Verification items for the finished model (mm, model axes). A direction names the side the tool comes from. Round coordinates to 2 decimals unless told otherwise and drop trailing zeros. Order: outer loops, then holes, each group sorted by start corner. A loop starts at its lowest first (then second) coordinate and runs counter-clockwise, first axis right, second up. Notation, with made-up numbers: (-31, -34) -> (15, -34) arc R14 cw to (15, -24) -> close; hole circle Ø4 at (36, 37). An arc over 180 degrees is marked (long way). Put each result on its own line as item: value.
```python
from build123d import *

# Parameters (mm, degrees)
BOSS_EXTRU_1_DEPTH      = 5
BOSS_EXTRU_1_2_DEPTH    = 5
BOSS_EXTRU_1_3_DEPTH    = 5
BOSS_EXTRU_1_4_DEPTH    = 5
BOSS_EXTRU_2_DEPTH      = 3
ENL_V_MAT_EXTRU_2_DEPTH = 186.027362841
ESQUISSE4_R             = 1.6
BOSS_EXTRU_3_DEPTH      = 3
BOSS_EXTRU_4_DEPTH      = 183.014563107
BOSS_EXTRU_6_DEPTH      = 169.006591337
BOSS_EXTRU_7_DEPTH      = 174.257281553
BOSS_EXTRU_8_DEPTH      = 177.5
ESQUISSE10_R            = 28
BOSS_EXTRU_9_DEPTH      = 2
BOSS_EXTRU_11_START     = 2.5
ESQUISSE11_W            = 257.5
ESQUISSE11_H            = 265.5
ESQUISSE11_R            = 28
BOSS_EXTRU_11_DEPTH     = 2.5
ESQUISSE12_R            = 2.1
BOSS_EXTRU_12_DEPTH     = 10.5
ESQUISSE13_R            = 5.1
ENL_V_MAT_EXTRU_3_DEPTH = 5
BOSS_EXTRU_13_DEPTH     = 10.5
ESQUISSE15_R            = 5.1
ENL_V_MAT_EXTRU_4_DEPTH = 5
CONG_1_R                = 1


with BuildPart() as part:
    # Esquisse1 → Boss.-Extru.1 (new body)
    with BuildSketch(Plane.XY):
        Polygon((128.75, -132.75), (88.75, -132.75), (88.75, -111.507281553), (108.75, -91.507281553), (128.75, -91.507281553), align=None)
    extrude(amount=BOSS_EXTRU_1_DEPTH)



with BuildPart() as body_2:
    # Esquisse1 → Boss.-Extru.1 2 (new body)
    with BuildSketch(Plane.XY):
        Polygon((128.75, 132.75), (80.256591337, 132.75), (80.256591337, 102.75), (100.256591337, 82.75), (128.75, 82.75), align=None)
    extrude(amount=BOSS_EXTRU_1_2_DEPTH)


with BuildPart() as body_3:
    # Esquisse1 → Boss.-Extru.1 3 (new body)
    with BuildSketch(Plane.XY):
        Polygon((-128.75, -132.75), (-128.75, -91.507281553), (-108.75, -91.507281553), (-88.75, -111.507281553), (-88.75, -132.75), align=None)
    extrude(amount=BOSS_EXTRU_1_3_DEPTH)


with BuildPart() as body_4:
    # Esquisse1 → Boss.-Extru.1 4 (new body)
    with BuildSketch(Plane.XY):
        Polygon((-88.75, 132.75), (-88.75, 111.507281553), (-108.75, 91.507281553), (-128.75, 91.507281553), (-128.75, 132.75), align=None)
    extrude(amount=BOSS_EXTRU_1_4_DEPTH)


with BuildPart() as part_1:
    add(part.part)

    add(body_2.part)  # Boss.-Extru.2 merges body 2

    add(body_3.part)  # Boss.-Extru.2 merges body 3

    add(body_4.part)  # Boss.-Extru.2 merges body 4
    # Esquisse2 → Boss.-Extru.2 (add)
    with BuildSketch(Plane(origin=(0, 0, 0), x_dir=(-1, 0, 0), z_dir=(0, 0, -1))):
        Polygon((-80.256591337, 127.75), (-80.256591337, 132.75), (-128.75, 132.75), (-128.75, 82.75), (-123.75, 82.75), (-123.75, 127.75), align=None)
        Polygon((-123.75, -127.75), (-88.75, -127.75), (-88.75, -132.75), (-128.75, -132.75), (-128.75, -91.507281553), (-123.75, -91.507281553), align=None)
        Polygon((88.75, -127.75), (88.75, -132.75), (128.75, -132.75), (128.75, -91.507281553), (123.75, -91.507281553), (123.75, -127.75), align=None)
        Polygon((128.75, 132.75), (88.75, 132.75), (88.75, 127.75), (123.75, 127.75), (123.75, 91.507281553), (128.75, 91.507281553), align=None)
    extrude(amount=BOSS_EXTRU_2_DEPTH)

    # Esquisse3 → Enlèv. mat.-Extru.2 (cut, through all)
    with BuildSketch(Plane.XY.offset(3)):
        Polygon((110, 82.75), (110, 110), (80.256591337, 110), (80.256591337, 102.75), (100.256591337, 82.75), align=None)
        Polygon((-90.257281553, 110), (-110, 110), (-110, 91.507281553), (-108.75, 91.507281553), align=None)
        Polygon((-110, -110), (-110, -91.507281553), (-108.75, -91.507281553), (-90.257281553, -110), align=None)
        Polygon((110, -91.507281553), (110, -110), (90.257281553, -110), (108.75, -91.507281553), align=None)
    extrude(amount=-ENL_V_MAT_EXTRU_2_DEPTH, mode=Mode.SUBTRACT)

    # Esquisse4 → Boss.-Extru.3 (add)
    with BuildSketch(Plane(origin=(0, 0, 3), x_dir=(-1, 0, 0), z_dir=(0, 0, -1))):
        with Locations(Location((-107.5, 107.5, 0), (0, 0, 180))):
            Circle(ESQUISSE4_R)
        with Locations((-107.5, -107.5)):
            Circle(ESQUISSE4_R)
        with Locations(Location((107.5, -107.5, 0), (0, 0, 180))):
            Circle(ESQUISSE4_R)
        with Locations(Location((107.5, 107.5, 0), (0, 0, 180))):
            Circle(ESQUISSE4_R)
    extrude(amount=BOSS_EXTRU_3_DEPTH)

    # Esquisse5 → Boss.-Extru.4 (add)
    with BuildSketch(Plane.XZ.offset(-91.507281553)):
        Polygon((-123.75, 0), (-110, 0), (-110, 3), (-108.75, 3), (-108.75, 5), (-128.75, 5), (-128.75, -3), (-123.75, -3), align=None)
    extrude(amount=BOSS_EXTRU_4_DEPTH)

    # Esquisse7 → Boss.-Extru.6 (add)
    with BuildSketch(Plane(origin=(-88.75, 0, 0), x_dir=(0, 0, -1), z_dir=(1, 0, 0))):
        Polygon((0, 111.507281553), (0, 127.75), (3, 127.75), (3, 132.75), (-5, 132.75), (-5, 111.507281553), align=None)
    extrude(amount=BOSS_EXTRU_6_DEPTH)

    # Esquisse8 → Boss.-Extru.7 (add)
    with BuildSketch(Plane(origin=(0, -91.507281553, 0), x_dir=(1, 0, 0), z_dir=(0, 1, 0))):
        Polygon((123.75, 0), (110, 0), (110, -3), (108.75, -3), (108.75, -5), (128.75, -5), (128.75, 3), (123.75, 3), align=None)
    extrude(amount=BOSS_EXTRU_7_DEPTH)

    # Esquisse9 → Boss.-Extru.8 (add)
    with BuildSketch(Plane.ZY.offset(-88.75)):
        Polygon((0, -111.507281553), (0, -127.75), (-3, -127.75), (-3, -132.75), (5, -132.75), (5, -111.507281553), align=None)
    extrude(amount=BOSS_EXTRU_8_DEPTH)

    # Esquisse10 → Boss.-Extru.9 (add)
    with BuildSketch(Plane.XY.offset(5)):
        with BuildLine():
            Line((100.256591337, 82.75), (31.902373727, 14.39578239))
            ThreePointArc((31.902373727, 14.39578239), (34.999858189, -0.099633105), (31.819897219, -14.577178773))
            Line((31.819897219, -14.577178773), (108.75, -91.507281553))
            Line((108.75, -91.507281553), (88.75, -111.507281553))
            Line((88.75, -111.507281553), (10.599223862, -33.356505415))
            ThreePointArc((10.599223862, -33.356505415), (0, -35), (-10.599223862, -33.356505415))
            Line((-10.599223862, -33.356505415), (-88.75, -111.507281553))
            Line((-88.75, -111.507281553), (-108.75, -91.507281553))
            Line((-108.75, -91.507281553), (-31.819897219, -14.577178773))
            ThreePointArc((-31.819897219, -14.577178773), (-35, 0), (-31.819897219, 14.577178773))
            Line((-31.819897219, 14.577178773), (-108.75, 91.507281553))
            Line((-108.75, 91.507281553), (-90.257281553, 110))
            Line((-90.257281553, 110), (-12.823491891, 32.566210337))
            ThreePointArc((-12.823491891, 32.566210337), (-1.075408771, 34.983474613), (10.798967391, 33.292376054))
            Line((10.798967391, 33.292376054), (80.256591337, 102.75))
            Line((80.256591337, 102.75), (100.256591337, 82.75))
        make_face()
        Circle(ESQUISSE10_R, mode=Mode.SUBTRACT)
    extrude(amount=-BOSS_EXTRU_9_DEPTH)

    # Esquisse11 → Boss.-Extru.11 (add)
    with BuildSketch(Plane.XY.offset(5).offset(BOSS_EXTRU_11_START)):
        Rectangle(ESQUISSE11_W, ESQUISSE11_H)
        Circle(ESQUISSE11_R, mode=Mode.SUBTRACT)
        with BuildLine():
            Line((80.256591337, 111.507281553), (80.256591337, 102.75))
            Line((80.256591337, 102.75), (10.798967391, 33.292376054))
            ThreePointArc((10.798967391, 33.292376054), (-1.075408771, 34.983474613), (-12.823491891, 32.566210337))
            Line((-12.823491891, 32.566210337), (-90.257281553, 110))
            Line((-90.257281553, 110), (-88.75, 111.507281553))
            Line((-88.75, 111.507281553), (80.256591337, 111.507281553))
        make_face(mode=Mode.SUBTRACT)
        with BuildLine():
            Line((-108.75, 91.507281553), (-31.819897219, 14.577178773))
            ThreePointArc((-31.819897219, 14.577178773), (-35, 0), (-31.819897219, -14.577178773))
            Line((-31.819897219, -14.577178773), (-108.75, -91.507281553))
            Line((-108.75, -91.507281553), (-108.75, 91.507281553))
        make_face(mode=Mode.SUBTRACT)
        with BuildLine():
            Line((-88.75, -111.507281553), (-10.599223862, -33.356505415))
            ThreePointArc((-10.599223862, -33.356505415), (0, -35), (10.599223862, -33.356505415))
            Line((10.599223862, -33.356505415), (88.75, -111.507281553))
            Line((88.75, -111.507281553), (-88.75, -111.507281553))
        make_face(mode=Mode.SUBTRACT)
        with BuildLine():
            Line((108.75, -91.507281553), (31.819897219, -14.577178773))
            ThreePointArc((31.819897219, -14.577178773), (34.999858189, -0.099633105), (31.902373727, 14.39578239))
            Line((31.902373727, 14.39578239), (100.256591337, 82.75))
            Line((100.256591337, 82.75), (108.75, 82.75))
            Line((108.75, 82.75), (108.75, -91.507281553))
        make_face(mode=Mode.SUBTRACT)
    extrude(amount=-BOSS_EXTRU_11_DEPTH)

    # Esquisse12 → Boss.-Extru.12 (add)
    # profile 1 of 2: a face of its own
    with BuildSketch(Plane(origin=(0, 0, -3), x_dir=(-1, 0, 0), z_dir=(0, 0, -1))):
        with BuildLine():
            Line((109.25, -140.25), (109.25, -132.75))
            Line((109.25, -132.75), (94.25, -132.75))
            Line((94.25, -132.75), (94.25, -140.25))
            ThreePointArc((94.25, -140.25), (101.75, -147.75), (109.25, -140.25))
        make_face()
        with Locations((101.75, -140.25)):
            Circle(ESQUISSE12_R, mode=Mode.SUBTRACT)
    # profile 2 of 2: a face of its own
    with BuildSketch(Plane(origin=(0, 0, -3), x_dir=(-1, 0, 0), z_dir=(0, 0, -1))):
        with BuildLine():
            Line((-110.75, -140.25), (-110.75, -132.75))
            Line((-110.75, -132.75), (-125.75, -132.75))
            Line((-125.75, -132.75), (-125.75, -140.25))
            ThreePointArc((-125.75, -140.25), (-118.25, -147.75), (-110.75, -140.25))
        make_face()
        with Locations((-118.25, -140.25)):
            Circle(ESQUISSE12_R, mode=Mode.SUBTRACT)
    extrude(amount=-BOSS_EXTRU_12_DEPTH)

    # Esquisse13 → Enlèv. mat.-Extru.3 (cut)
    with BuildSketch(Plane(origin=(0, 0, -3), x_dir=(-1, 0, 0), z_dir=(0, 0, -1))):
        with Locations((-118.25, -140.25)):
            Circle(ESQUISSE13_R)
        with Locations((101.75, -140.25)):
            Circle(ESQUISSE13_R)
    extrude(amount=-ENL_V_MAT_EXTRU_3_DEPTH, mode=Mode.SUBTRACT)

    # Esquisse14 → Boss.-Extru.13 (add)
    with BuildSketch(Plane(origin=(0, 0, -3), x_dir=(-1, 0, 0), z_dir=(0, 0, -1))):
        with BuildLine():
            Line((95, 134.75), (95, 132.75))
            Line((95, 132.75), (101.109687576, 132.75))
            ThreePointArc((101.109687576, 132.75), (100.51198871, 136.44626886), (103.85, 134.75))
            ThreePointArc((103.85, 134.75), (103.44626886, 133.51198871), (102.390312424, 132.75))
            Line((102.390312424, 132.75), (108.5, 132.75))
            Line((108.5, 132.75), (108.5, 134.75))
            ThreePointArc((108.5, 134.75), (101.75, 141.5), (95, 134.75))
        make_face()
        with BuildLine():
            ThreePointArc((-111.5, 134.75), (-118.25, 141.5), (-125, 134.75))
            Line((-125, 134.75), (-125, 132.75))
            Line((-125, 132.75), (-118.890312424, 132.75))
            ThreePointArc((-118.890312424, 132.75), (-119.48801129, 136.44626886), (-116.15, 134.75))
            ThreePointArc((-116.15, 134.75), (-116.55373114, 133.51198871), (-117.609687576, 132.75))
            Line((-117.609687576, 132.75), (-111.5, 132.75))
            Line((-111.5, 132.75), (-111.5, 134.75))
        make_face()
    extrude(amount=-BOSS_EXTRU_13_DEPTH)

    # Esquisse15 → Enlèv. mat.-Extru.4 (cut)
    with BuildSketch(Plane(origin=(0, 0, -3), x_dir=(-1, 0, 0), z_dir=(0, 0, -1))):
        with Locations((101.75, 134.75)):
            Circle(ESQUISSE15_R)
        with Locations((-118.25, 134.75)):
            Circle(ESQUISSE15_R)
    extrude(amount=-ENL_V_MAT_EXTRU_4_DEPTH, mode=Mode.SUBTRACT)

    # Congé1
    cong_1_edges = [part_1.edges().sort_by_distance(p)[0] for p in [
        (-109.1, 107.5, 0),
        (-109.1, -107.5, 0),
        (109.1, -107.5, 0),
    ]]
    fillet(cong_1_edges, radius=CONG_1_R)


solid = part_1.part
```
Item 1: Sectioned sample at B-B, the plane y = 98.5. Record the boundary of the cut face in (x, z).
Geometry check:
outline: (-128.75, -3) -> (-123.75, -3) -> (-123.75, 0) -> (-110, 0) -> (-110, 3) -> (-78.76, 3) -> (-78.76, 7.5) -> (-128.75, 7.5) -> close; (76.01, 3) -> (110, 3) -> (110, 0) -> (123.75, 0) -> (123.75, -3) -> (128.75, -3) -> (128.75, 7.5) -> (76.01, 7.5) -> close
Item 2: Depth check by flat-ended pin: pin 1 Ø6 at (x, z) = (22.5, -1) entering from -Y; pin 2 Ø2.5 at (x, y) = (108, 107.5) entering from -Z; pin 3 Ø4 at (x, z) = (-0.5, 5) entering from +Y. Enter the tip coordinate at first touch or a pass-through.
Geometry check:
pin 1: y = -132.75
pin 2: z = 0
pin 3: y = 132.75
Item 3: Tool access check on faces 1 (the face through (-50.22, -72.98, 5.28)), 2 (the face through (-101.7, 132.6, 2)), 3 (the face through (-119, -132.75, 2)), 4 (the face through (7, 132.75, 2)). Record the directions out of +Z, -Z, +X, -X, +Y, -Y that give a thin tool (end or side, any length) a straight path to the whole face; none if there is none.
Geometry check:
face 1: +Z, -Z
face 2: -Z
face 3: +Z, -Z, -X, -Y
face 4: +Z, -Z, +Y
Item 4: Sectioned sample at C-C, the plane x = -58. Record the boundary of the cut face in (y, z), then the cut area to 3 significant figures.
Geometry check:
outline: (-132.75, -3) -> (-127.75, -3) -> (-127.75, 0) -> (-111.51, 0) -> (-111.51, 7.5) -> (-132.75, 7.5) -> close; (-80.76, 3) -> (-40.76, 3) -> (-40.76, 7.5) -> (-80.76, 7.5) -> close; (40.76, 3) -> (77.74, 3) -> (77.74, 7.5) -> (40.76, 7.5) -> close; (111.51, 0) -> (127.75, 0) -> (127.75, -3) -> (132.75, -3) -> (132.75, 7.5) -> (111.51, 7.5) -> close
area: 695 mm2
Item 5: Sectioned sample at A-A, the plane y = 0. Record the boundary of the cut face in (x, z), then the cut area to 4 significant figures.
Geometry check:
outline: (-128.75, -3) -> (-123.75, -3) -> (-123.75, 0) -> (-110, 0) -> (-110, 3) -> (-108.75, 3) -> (-108.75, 7.5) -> (-128.75, 7.5) -> close; (-35, 3) -> (-28, 3) -> (-28, 7.5) -> (-35, 7.5) -> close; (28, 3) -> (35, 3) -> (35, 7.5) -> (28, 7.5) -> close; (108.75, 3) -> (110, 3) -> (110, 0) -> (123.75, 0) -> (123.75, -3) -> (128.75, -3) -> (128.75, 7.5) -> (108.75, 7.5) -> close
area: 385.5 mm2
Item 6: Sectioned sample at D-D, the plane z = 5. Give the number of separate pieces and of enclosed holes in the cut face, then the cut area to 3 significant figures.
Geometry check:
separate pieces: 1
enclosed holes: 9
area: 34,600 mm2
Item 7: Material ranges on line 1 along X through (y, z) = (-140.25, 4.2); line 2 along Y through (x, z) = (118.25, 0.9); line 3 along X through (y, z) = (-42.5, 1), recorded low to high.
Geometry check:
line 1: -109.25 to -103.85, -99.65 to -94.25, 110.75 to 116.15, 120.35 to 125.75
line 2: -147.75 to -145.35, -135.15 to 129.65, 139.85 to 141.5
line 3: -128.75 to -110, 110 to 128.75
Item 8: Release check for a two-part mould opening along Y. For faces 5 (the face through (7, -132.75, 2)), 6 (the face through (123.345, -140.026, -0.535)), 7 (the face through (80.257, 108, 5)), 8 (the face through (118.1, 141.5, 2.2)) record: pulls with the +Y half, pulls with the -Y half, needs draft (parallel to the pull), parting line crosses it, or undercut.
Geometry check:
face 5: pulls with the -Y half
face 6: undercut
face 7: undercut
face 8: pulls with the +Y half
